from build123d import *

# Parameters (mm, degrees)
F1_DEPTH  = 3.2
F3_COUNT  = 3
F4_R      = 4.175
F5_DEPTH  = 1
F6_R      = 3.175
F7_DEPTH  = 1.5
F8_R      = 1.95
F9_DEPTH  = 5.7
F10_R     = 6.4
F11_DEPTH = 25
F12_R     = 5
F13_SIZE  = 1


with BuildPart() as f1:
    # F0 (on Top) → F1 (new body)
    with BuildSketch(Plane.XY):
        with BuildLine():
            Line((-3, 8.9084229805), (-3, 19))
            ThreePointArc((-3, 19), (0, 18), (3, 19))
            Line((3, 19), (3, 8.9084229805))
            ThreePointArc((3, 8.9084229805), (4.0280174031, 8.4932370625), (5, 7.9598994969))
            Line((5, 7.9598994969), (5, 23))
            ThreePointArc((5, 23), (0, 28), (-5, 23))
            Line((-5, 23), (-5, 7.9598994969))
            ThreePointArc((-5, 7.9598994969), (-4.0280174031, 8.4932370625), (-3, 8.9084229805))
        make_face()
        with BuildLine():
            Line((-3, 7.5055534995), (-3, 8.9084229805))
            ThreePointArc((-3, 8.9084229805), (-4.0280174031, 8.4932370625), (-5, 7.9598994969))
            Line((-5, 7.9598994969), (-5, 2.8867513459))
            Line((-5, 2.8867513459), (0, 0))
            Line((0, 0), (5, 2.8867513459))
            Line((5, 2.8867513459), (5, 7.9598994969))
            ThreePointArc((5, 7.9598994969), (4.0280174031, 8.4932370625), (3, 8.9084229805))
            Line((3, 8.9084229805), (3, 7.5055534995))
            Line((3, 7.5055534995), (0, 5.7735026919))
            Line((0, 5.7735026919), (-3, 7.5055534995))
        make_face()
        with BuildLine():
            Line((-5, 2.8867513459), (-5, 7.9598994969))
            ThreePointArc((-5, 7.9598994969), (-4.5475268004, -8.2267855205), (9.4, 0))
            ThreePointArc((9.4, 0), (8.2267855205, 4.5475268004), (5, 7.9598994969))
            Line((5, 7.9598994969), (5, 2.8867513459))
            Line((5, 2.8867513459), (0, 0))
            Line((0, 0), (-5, 2.8867513459))
        make_face()
    extrude(amount=F1_DEPTH)

    # F3: F1 ×3 about axis
    f3_axis = Axis((0, 0, 19.5818599313), (0, 0, 1))


with BuildPart() as f1_1:
    add(f1.part)
    for i in range(1, F3_COUNT):
        add(f1.part.rotate(f3_axis, i * 360 / F3_COUNT))

    # F4 (on face) → F5 (join)
    with BuildSketch(Plane.XY.offset(3.2)):
        with Locations((0, 23)):
            Circle(F4_R)
        with Locations((-19.918584287, -11.5)):
            Circle(F4_R)
        with Locations((19.918584287, -11.5)):
            Circle(F4_R)
    extrude(amount=F5_DEPTH)

    # F6 (on face) → F7 (join)
    with BuildSketch(Plane.XY.offset(4.2)):
        with Locations((0, 23)):
            Circle(F6_R)
        with Locations((-19.918584287, -11.5)):
            Circle(F6_R)
        with Locations((19.918584287, -11.5)):
            Circle(F6_R)
    extrude(amount=F7_DEPTH)

    # F8 (on face) → F9 (cut, through all)
    with BuildSketch(Plane.XY.offset(5.7)):
        with Locations((0, 23)):
            Circle(F8_R)
        with Locations((-19.918584287, -11.5)):
            Circle(F8_R)
        with Locations((19.918584287, -11.5)):
            Circle(F8_R)
    extrude(amount=-F9_DEPTH, mode=Mode.SUBTRACT)

    # F10 (on face) → F11 (cut)
    with BuildSketch(Plane.XY.offset(3.2)):
        Circle(F10_R)
    extrude(amount=-F11_DEPTH, mode=Mode.SUBTRACT)

    # F12
    f12_edges = [f1_1.edges().sort_by_distance(p)[0] for p in [
        (-5, 7.959899, 1.6),
        (-9.393475, 0.350177, 1.6),
        (-4.393475, -8.310077, 1.6),
        (4.393475, -8.310077, 1.6),
        (9.393475, 0.350177, 1.6),
        (5, 7.959899, 1.6),
    ]]
    fillet(f12_edges, radius=F12_R)

    # F13
    f13_edges = [f1_1.edges().sort_by_distance(p)[0] for p in [
        (-24.248711, -14, 0),
    ]]
    chamfer(f13_edges, length=F13_SIZE)


solid = f1_1.part
Could you check a few things on this model? Use its own coordinates, in mm. A direction names the side the tool comes from. Round coordinates to 2 decimals unless told otherwise and drop trailing zeros. Write each loop counter-clockwise with the first axis right and the second up, starting at its lowest first coordinate (ties: lowest second). Pieces come first, ordered by that corner, then holes. Notation, with made-up numbers: (-19, 17) - (-4, 17) arc R23 ccw to (-4, 34) - close; hole circle Ø1 at (24, 55.25). An arc over 180 degrees is marked (long way). Put each result on its own line as item: value. Start each with the question number.
(1) Will these pins go through, and if not, where does the flat tip stop? pin 1 (1 mm diameter, centred on x = 16.5, z = 4.5, fed in from +Y); pin 2 (3.5 mm diameter, centred on x = 0, y = 23, fed in from -Z); pin 3 (2.5 mm diameter, centred on y = 15.5, z = 2, fed in from -X); pin 4 (1 mm diameter, centred on y = -10.5, z = 3.5, fed in from -X).
(2) I need wall thicknesses on probe 1 along Y at (x, z) = (0, 1.6); probe 2 along X at (y, z) = (16.5, 1.65); probe 3 along Z at (x, y) = (-6, 5.5). Which ranges of each line are inside material? Lowest first, please.
(3) I want a section at A-A, the plane x = 0. Please give me the cut outline in (y, z) (3 decimals).
(4) I want a section at C-C, the plane z = 1.7. Give the number of separate pieces and of enclosed holes in the cut face, plus the area to 3 significant figures.
(5) I want a section at B-B, the plane y = 15. Please give me the cut outline in (x, z), plus the area to 3 significant figures.
(6) Thinking about a two-plate mould opening in X: for faces 6 (the flat face through (5, 17, 2)), 7 (the cylindrical face through (21.72, -12.25, 2.89)), 8 (the flat face through (18, -13, 5.7)), 9 (the flat face through (-5, 17, 2)), which applies, released by +X, released by -X, zero draft, split by the parting line, or undercut?
(7) For faces 1 (the flat face through (-12, -12.7, 2.1)), 2 (the cylindrical face through (22.85, -12.72, 4.94)), 3 (the flat face through (-20, -14, 5.7)), 4 (the flat face through (3, 14, 2)), 5 (the cylindrical face through (-9.963, 0.494, 2.115)), which set-ups out of +Z, -Z, +X, -X, +Y, -Y let a thin tool reach every point of the face, with its end or its side?
Here are the results:
1. pin 1: stops at y = -8.62
1. pin 2: passes through
1. pin 3: stops at x = -5
1. pin 4: stops at x = -24.88
2. probe 1: y = -9.4 to -6.4, 6.4 to 9.4, 18 to 21.05, 24.95 to 28
2. probe 2: x = -5 to -3, 3 to 5
2. probe 3: z = 0 to 3.2
3. outline: (-9.4, 1) - (-8.4, 0) - (-6.4, 0) - (-6.4, 3.2) - (-9.4, 3.2) - close; (6.4, 0) - (9.4, 0) - (9.4, 3.2) - (6.4, 3.2) - close; (18, 0) - (21.05, 0) - (21.05, 5.7) - (19.825, 5.7) - (19.825, 4.2) - (18.825, 4.2) - (18.825, 3.2) - (18, 3.2) - close; (24.95, 0) - (27, 0) - (28, 1) - (28, 3.2) - (27.175, 3.2) - (27.175, 4.2) - (26.175, 4.2) - (26.175, 5.7) - (24.95, 5.7) - close
4. separate pieces: 1
4. enclosed holes: 7
4. area: 494 mm^2
5. outline: (-5, 1) - (-4, 0) - (-3, 0) - (-3, 3.2) - (-5, 3.2) - close; (3, 0) - (4, 0) - (5, 1) - (5, 3.2) - (3, 3.2) - close
5. area: 11.8 mm^2
6. face 6: released by +X
6. face 7: undercut
6. face 8: zero draft
6. face 9: released by -X
7. face 1: +Z, -Z, -Y
7. face 2: +Z
7. face 3: +Z, +X, -X, +Y, -Y
7. face 4: +Z, -Z
7. face 5: +Z, -Z, -X, +Y
